```python
from build123d import *

# Parameters (mm, degrees)
SKETCH1_W           = 5.5
SKETCH1_H           = 20.5
BOSS_EXTRUDE1_DEPTH = 2.5


with BuildPart() as part:
    # Sketch1 → Boss-Extrude1 (new, symmetric)
    with BuildSketch(Plane.XY):
        Polygon((143.545659386, -48.941167375), (143.545659386, -53.941167375), (103.795659386, -53.941167375), (103.795659386, -64.191167375), (98.295659386, -64.191167375), (98.295659386, -53.941167375), (93.545659386, -53.941167375), (93.545659386, -48.941167375), (83.545659386, -48.941167375), (83.545659386, -103.691167375), (93.795659386, -103.691167375), (93.795659386, -109.191167375), (83.545659386, -109.191167375), (83.545659386, -128.691167375), (93.795659386, -128.691167375), (93.795659386, -134.191167375), (83.545659386, -134.191167375), (83.545659386, -153.691167375), (93.795659386, -153.691167375), (93.795659386, -159.191167375), (83.545659386, -159.191167375), (83.545659386, -213.941167375), (93.545659386, -213.941167375), (93.545659386, -208.941167375), (98.295659386, -208.941167375), (98.295659386, -198.691167375), (103.795659386, -198.691167375), (103.795659386, -208.941167375), (143.545659386, -208.941167375), (143.545659386, -213.941167375), (163.545659386, -213.941167375), (163.545659386, -208.941167375), (203.295659386, -208.941167375), (203.295659386, -198.691167375), (208.795659386, -198.691167375), (208.795659386, -208.941167375), (213.545659386, -208.941167375), (213.545659386, -213.941167375), (223.545659386, -213.941167375), (223.545659386, -159.191167375), (213.295659386, -159.191167375), (213.295659386, -153.691167375), (223.545659386, -153.691167375), (223.545659386, -134.191167375), (213.295659386, -134.191167375), (213.295659386, -128.691167375), (223.545659386, -128.691167375), (223.545659386, -109.191167375), (213.295659386, -109.191167375), (213.295659386, -103.691167375), (223.545659386, -103.691167375), (223.545659386, -48.941167375), (213.545659386, -48.941167375), (213.545659386, -53.941167375), (208.795659386, -53.941167375), (208.795659386, -64.191167375), (203.295659386, -64.191167375), (203.295659386, -53.941167375), (163.545659386, -53.941167375), (163.545659386, -48.941167375), align=None)
        with Locations((101.045659386, -131.441167375)):
            Rectangle(SKETCH1_W, SKETCH1_H, mode=Mode.SUBTRACT)
        with Locations((206.045659386, -131.441167375)):
            Rectangle(SKETCH1_W, SKETCH1_H, mode=Mode.SUBTRACT)
        with Locations((176.045659386, -131.441167375)):
            Rectangle(SKETCH1_W, SKETCH1_H, mode=Mode.SUBTRACT)
        with Locations((131.045659386, -131.441167375)):
            Rectangle(SKETCH1_W, SKETCH1_H, mode=Mode.SUBTRACT)
    extrude(amount=BOSS_EXTRUDE1_DEPTH, both=True)


solid = part.part
```
The listing builds one solid part. Answer for the finished solid, in the listing's coordinates (mm). A direction names the side the tool comes from. Coordinates: 2 decimals unless noted, no trailing zeros. Order: outer loops, then holes, each group sorted by start corner. A loop starts at its lowest first (then second) coordinate and runs counter-clockwise, first axis right, second up. Notation, with made-up numbers: M 77,-34 L 123,-34 A20 cw 123,-23 Z; hole C 21.5,73 d6. An arc over 180 degrees is marked long. Answer as a JSON object with one key per item and string values. Group by question number.
1. Straight lines are drawn through the part: line 1 (Y direction, x = 217, z = -1.6); line 2 (X direction, y = -62, z = -1.75); line 3 (X direction, y = -141, z = -1.85). For each, find the intervals that lie inside material, in ascending order.
2. Determine the mould class of faces 4 (the flat face through (93.796, -156, 0)), 5 (the flat face through (89, -159.191, 0)), 6 (the flat face through (223.546, -187, 0)), 7 (the flat face through (203.296, -204, 0)) for opening direction X: released by +X, released by -X, zero draft, split by the parting line, or undercut.
3. Section B-B on y = -156 is taken. Write down the section's boundary in (x, z).
4. Section A-A on x = 109 is taken. Write down the section's boundary in (y, z), then the cut area to 3 significant figures.
5. A tool of negligible diameter and unlimited length cuts with its end or side. For faces 1 (the flat face through (101, -198.691, 0)), 2 (the flat face through (98.296, -59, 0)), 3 (the flat face through (103.796, -132, 0)), from which of +Z, -Z, +X, -X, +Y, -Y can it reach the whole face along a straight path? Write none if from no direction.
6. Section C-C on z = -0.85 is taken. State how many separate pieces and enclosed holes the cut face has, then the cut area to 3 significant figures.
7. Flat-ended cylindrical pins translate along their axes: P1, Ø1.5, axis at x = 131.5, y = -139.5, coming from the +Z side; P2, Ø2.5, axis at y = -156, z = 1, coming from the +X side; P3, Ø2, axis at x = 104.5, z = -1, coming from the +Y side. Find the tip coordinate at first contact, or state that the pin passes through.
Values follow:
{
 "1": {"line 1": "-213.94 to -159.19, -153.69 to -134.19, -128.69 to -109.19, -103.69 to -48.94", "line 2": "83.55 to 98.3, 103.8 to 203.3, 208.8 to 223.55", "line 3": "83.55 to 98.3, 103.8 to 128.3, 133.8 to 173.3, 178.8 to 203.3, 208.8 to 223.55"},
 "2": {"face 4": "released by -X", "face 5": "zero draft", "face 6": "released by +X", "face 7": "undercut"},
 "3": {"outline": "M 93.8,-2.5 L 213.3,-2.5 L 213.3,2.5 L 93.8,2.5 Z"},
 "4": {"outline": "M -208.94,-2.5 L -53.94,-2.5 L -53.94,2.5 L -208.94,2.5 Z", "area": "775 mm2"},
 "5": {"face 1": "+Z, -Z, -Y", "face 2": "+Z, -Z, +Y", "face 3": "+Z, -Z"},
 "6": {"separate pieces": "1", "enclosed holes": "4", "area": "21,100 mm2"},
 "7": {"P1": "through", "P2": "x = 213.3", "P3": "y = -53.94"}
}
